```python
from build123d import *

# Parameters (mm, degrees)
CHANFREIN1_SIZE         = 0.5
ENL_V_MAT_EXTRU_1_DEPTH = 2.3


with BuildPart() as part:
    # Esquisse1 → Révolution1 (revolve)
    with BuildSketch(Plane.XY):
        Polygon((0, 0), (0, 5), (0.5, 5), (3, 2.5), (16, 2.5), (16, 0), align=None)
    revolve(axis=Axis((16, 0, 0), (-1, 0, 0)))

    # Chanfrein1
    chanfrein1_edges = [part.edges().sort_by_distance(p)[0] for p in [
        (16, -2.5, 0),
    ]]
    chamfer(chanfrein1_edges, length=CHANFREIN1_SIZE)

    # Esquisse2 → Enlèv. mat.-Extru.1 (cut)
    with BuildSketch(Plane.ZY):
        Polygon((0, 1.732050808), (-1.5, 0.866025404), (-1.5, -0.866025404), (0, -1.732050808), (1.5, -0.866025404), (1.5, 0.866025404), align=None)
    extrude(amount=-ENL_V_MAT_EXTRU_1_DEPTH, mode=Mode.SUBTRACT)


solid = part.part
```
The model under review builds one solid part; all positions refer to its coordinate system, in mm. A direction names the side the tool comes from. Round coordinates to 2 decimals unless told otherwise and drop trailing zeros. Write each loop counter-clockwise with the first axis right and the second up, starting at its lowest first coordinate (ties: lowest second). Pieces come first, ordered by that corner, then holes. Notation, with made-up numbers: (-30, -20) - (1, -20) arc R33 cw to (1, 14) - close; hole circle Ø2 at (55, -29). An arc over 180 degrees is marked (long way). Answer as CSV lines item,"result". Start each with the question number.
(1) We need section B-B on x = 7.25. State the section outline as (y, z) points.
(2) For faces 4 (the flat face through (1.134, -1.293, -0.76)), 5 (the cylindrical face through (9.34, -0.54, 2.44)), 6 (the flat face through (16, 0, 0)), list the 3-axis set-ups (+Z, -Z, +X, -X, +Y, -Y) from which the entire face can be reached by the end or side of a thin tool; tool diameter is ignored.
(3) We need section A-A on y = 0. State the section outline as (x, z) points.
(4) To check wall thickness, follow line 1 (Y direction, x = 8.25, z = 1.5); line 2 (X direction, y = 1, z = 0.25); line 3 (Y direction, x = 3.5, z = 2). State the ranges of each line that lie inside material, in increasing order.
(5) Draft analysis for pull direction Y (two halves, no side actions). For faces 1 (the flat face through (0, 0, 2)), 2 (the cylindrical face through (0.25, -1.08, 4.88)), 3 (the flat face through (1, 0, 1.5)), state which applies: pulls with the +Y half, pulls with the -Y half, needs draft (parallel to the pull), parting line crosses it, or undercut.
(6) For pin 1 Ø1.5 at (x, z) = (9.5, 1.5) entering from -Y; pin 2 Ø1.5 at (x, z) = (6.5, -0.5) entering from +Y; pin 3 Ø1.5 at (y, z) = (0.5, -0.5) entering from -X, all flat-tipped, find the tip position at first contact; note any pin that passes through.
Worked answers:
1,outline,"circle Ø5 at (0, 0)"
2,face 4,"-X"
2,face 5,"+X"
2,face 6,"+Z, -Z, +X, +Y, -Y"
3,outline,"(0, -5) - (0.5, -5) - (3, -2.5) - (15.5, -2.5) - (16, -2) - (16, 2) - (15.5, 2.5) - (3, 2.5) - (0.5, 5) - (0, 5) - (0, 1.5) - (2.3, 1.5) - (2.3, -1.5) - (0, -1.5) - close"
4,line 1,"-2 to 2"
4,line 2,"2.3 to 16"
4,line 3,"-1.5 to 1.5"
5,face 1,"needs draft"
5,face 2,"parting line crosses it"
5,face 3,"undercut"
6,pin 1,"y = -2.38"
6,pin 2,"y = 2.5"
6,pin 3,"x = 2.3"
